Build history of the part. All positions in model axes, mm. A direction names the side the tool comes from. Give positions to 0.01 mm unless a question says otherwise; leave off trailing zeros. Order: outer loops, then holes, each group sorted by start corner. A loop starts at its lowest first (then second) coordinate and runs counter-clockwise, first axis right, second up. Notation, with made-up numbers: (61.5, 12.5) -> (68.5, 12.5) arc R8 cw to (68.5, 16.5) -> close; hole circle Ø5 at (-31, 59). An arc over 180 degrees is marked (long way). Write item = value, one per line. Start each with the question number.
from build123d import *

# Parameters (mm, degrees)
SKETCH2_R         = 1.4224
EXTRUDE1_DEPTH    = 4.7625
CHAMFER1_SIZE     = 0.47625
EXTRUDE4_DEPTH    = 9.525
SKETCH8_OUTSIDE_W = 62.926
SKETCH8_OUTSIDE_H = 63.664
SKETCH8_OUTSIDE_R = 2.38125
EXTRUDE5_DEPTH    = 15.2875
EXTRUDE5_TAPER    = 60
SKETCH9_OUTSIDE_W = 46.428
SKETCH9_OUTSIDE_H = 47.166
SKETCH9_OUTSIDE_R = 2.38125
EXTRUDE6_DEPTH    = 10.525
EXTRUDE6_TAPER    = 60
SKETCH10_R        = 1.4224
EXTRUDE7_DEPTH    = 6.35


with BuildPart() as part:
    # Sketch2 → Extrude1 (new body)
    with BuildSketch(Plane(origin=(7.14375, 0, 0), x_dir=(0, 0, -1), z_dir=(1, 0, 0))):
        Circle(SKETCH2_R)
    extrude(amount=-EXTRUDE1_DEPTH)

    # Chamfer1
    chamfer1_edges = [part.edges().sort_by_distance(p)[0] for p in [
        (7.14375, 0, 1.4224),
    ]]
    chamfer(chamfer1_edges, length=CHAMFER1_SIZE)

    # Sketch7 → Extrude4 (add)
    with BuildSketch(Plane(origin=(2.38125, 0, 0), x_dir=(0, 0, -1), z_dir=(1, 0, 0))):
        Polygon((0, 2.749630657), (-2.38125, 1.374815329), (-2.38125, -1.374815329), (0, -2.749630657), (2.38125, -1.374815329), (2.38125, 1.374815329), align=None)
    extrude(amount=-EXTRUDE4_DEPTH)

    # Sketch8 outside → Extrude5 (cut, through all)
    with BuildSketch(Plane.ZY.offset(7.14375)):
        Rectangle(SKETCH8_OUTSIDE_W, SKETCH8_OUTSIDE_H)
        Circle(SKETCH8_OUTSIDE_R, mode=Mode.SUBTRACT)
    extrude(amount=-EXTRUDE5_DEPTH, taper=EXTRUDE5_TAPER, mode=Mode.SUBTRACT)

    # Sketch9 outside → Extrude6 (cut, through all)
    with BuildSketch(Plane(origin=(2.38125, 0, 0), x_dir=(0, 0, -1), z_dir=(1, 0, 0))):
        Rectangle(SKETCH9_OUTSIDE_W, SKETCH9_OUTSIDE_H)
        Circle(SKETCH9_OUTSIDE_R, mode=Mode.SUBTRACT)
    extrude(amount=-EXTRUDE6_DEPTH, taper=EXTRUDE6_TAPER, mode=Mode.SUBTRACT)

    # Sketch10 → Extrude7 (cut)
    with BuildSketch(Plane.ZY.offset(7.14375)):
        Circle(SKETCH10_R)
    extrude(amount=-EXTRUDE7_DEPTH, mode=Mode.SUBTRACT)


solid = part.part
(1) Cut at A-A, the plane x = -3.25. Give the cut face in (y, z).
(2) Cut at C-C, the plane x = 1.75. Give the cut face in (y, z).
(3) 3-axis set-ups, long thin cutter, end or side, ignore diameter. For faces 1 (the face through (2.381, -2, 0)), 2 (the face through (-7.07, -1.25, 2.18)): which of +Z, -Z, +X, -X, +Y, -Y reach the whole face in a straight line?
(4) Wall check: line 1 (Z direction, x = -5, y = -0.1); line 2 (X direction, y = -1.6, z = -0.3); line 3 (Z direction, x = -2.25, y = 0.6). Give the ranges that are in metal, low to high. Write a range as [from, to].
(5) Cut at B-B, the plane x = 3.75. Give the cut face in (y, z).
(6) Flat gauge pins, fed straight in: P1, Ø0.9, axis at y = 0, z = 0, coming from the -X side; P2, Ø1.5, axis at x = 3.5, y = 1.5, coming from the -Z side. Where does each tip first touch, or does it go through?
(7) Mould opens along Z. For faces 3 (the face through (-2.315, -2.072, -1.174)), 4 (the face through (-0.794, 0, 0)), 5 (the face through (-4.01, -1.39, -0.31)), 6 (the face through (4.55, -1.39, 0.31)) say: released by +Z, released by -Z, zero draft, split by the parting line, or undercut.
Results:
q1.outline = (-2.75, 0) -> (-1.37, -2.38) -> (1.37, -2.38) -> (2.75, 0) -> (1.37, 2.38) -> (-1.37, 2.38) -> close; hole circle Ø2.84 at (0, 0)
q2.outline = (-2.75, 0) -> (-1.37, -2.38) -> (1.37, -2.38) -> (2.75, 0) -> (1.37, 2.38) -> (-1.37, 2.38) -> close
q3.face_1 = +X
q3.face_2 = +Z, -X, -Y
q4.line_1 = [-2.38, -1.42], [1.42, 2.38]
q4.line_2 = [-7.14, 2.38]
q4.line_3 = [-2.38, -1.29], [1.29, 2.38]
q5.outline = circle Ø2.84 at (0, 0)
q6.P1 = -0.79
q6.P2 = -1.21
q7.face_3 = released by -Z
q7.face_4 = undercut
q7.face_5 = undercut
q7.face_6 = split by the parting line
